Part model, mm, in its own coordinate system. Face numbers are marked on the shaded views. A direction names the side the tool comes from. Give positions to 0.01 mm unless a question says otherwise; leave off trailing zeros. Loops run counter-clockwise (first coordinate to the right, second up) from the corner with the lowest first, then second, coordinate; pieces in that order, holes last. Notation, with made-up numbers: M -35.75,-35 L 8.25,-35 A20 ccw 8.25,-28 Z; hole C 17.25,89 d2. An arc over 180 degrees is marked long. Put each result on its own line as item: value. Start each with the question number.
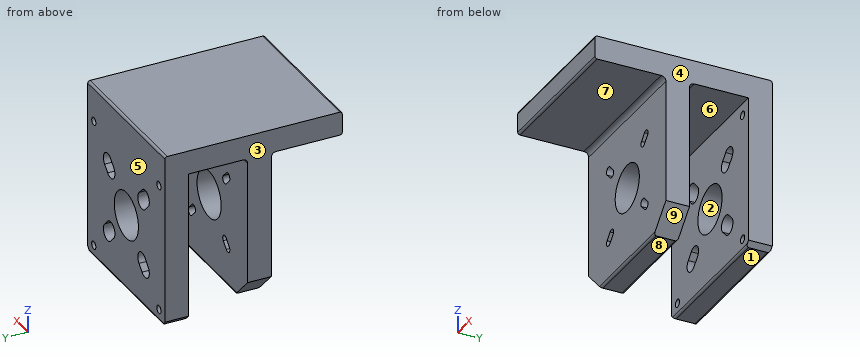
```python
from build123d import *

# Parameters (mm, degrees)
SKETCH_W        = 64
SKETCH_H        = 64
SKETCH_R        = 10
SKETCH_R_2      = 1.7
PAD_DEPTH       = 10
SKETCH001_W     = 64
SKETCH001_H     = 35
PAD001_DEPTH    = 10
SKETCH002_W     = 64
SKETCH002_H     = 74
SKETCH002_R     = 10
PAD002_DEPTH    = 10
SKETCH003_W     = 64
SKETCH003_H     = 10
PAD003_DEPTH    = 30
CHAMFER_SIZE    = 2
CHAMFER001_SIZE = 10
FILLET_R        = 2
FILLET001_R     = 1


with BuildPart() as part:
    # Sketch → Pad (new body)
    with BuildSketch(Plane.XZ):
        Rectangle(SKETCH_W, SKETCH_H)
        Circle(SKETCH_R, mode=Mode.SUBTRACT)
        with Locations((27, 27)):
            Circle(SKETCH_R_2, mode=Mode.SUBTRACT)
        with Locations((-27, -27)):
            Circle(SKETCH_R_2, mode=Mode.SUBTRACT)
        with Locations((-27, 27)):
            Circle(SKETCH_R_2, mode=Mode.SUBTRACT)
        with Locations((27, -27)):
            Circle(SKETCH_R_2, mode=Mode.SUBTRACT)
        with BuildLine():
            ThreePointArc((10.525126, 15.474874), (10.525126, 10.525126), (15.474874, 10.525126))
            Line((17.974874, 13.025126), (15.474874, 10.525126))
            ThreePointArc((17.974874, 13.025126), (17.974874, 17.974874), (13.025126, 17.974874))
            Line((13.025126, 17.974874), (10.525126, 15.474874))
        make_face(mode=Mode.SUBTRACT)
        with BuildLine():
            ThreePointArc((-13.025126, 17.974874), (-17.974874, 17.974874), (-17.974874, 13.025126))
            Line((-15.474874, 10.525126), (-17.974874, 13.025126))
            ThreePointArc((-15.474874, 10.525126), (-10.525126, 10.525126), (-10.525126, 15.474874))
            Line((-10.525126, 15.474874), (-13.025126, 17.974874))
        make_face(mode=Mode.SUBTRACT)
        with BuildLine():
            ThreePointArc((13.025126, -17.974874), (17.974874, -17.974874), (17.974874, -13.025126))
            Line((15.474874, -10.525126), (17.974874, -13.025126))
            ThreePointArc((15.474874, -10.525126), (10.525126, -10.525126), (10.525126, -15.474874))
            Line((10.525126, -15.474874), (13.025126, -17.974874))
        make_face(mode=Mode.SUBTRACT)
        with BuildLine():
            ThreePointArc((-17.974874, -13.025126), (-17.974874, -17.974874), (-13.025126, -17.974874))
            Line((-10.525126, -15.474874), (-13.025126, -17.974874))
            ThreePointArc((-10.525126, -15.474874), (-10.525126, -10.525126), (-15.474874, -10.525126))
            Line((-15.474874, -10.525126), (-17.974874, -13.025126))
        make_face(mode=Mode.SUBTRACT)
    extrude(amount=PAD_DEPTH)

    # Sketch001 (on Face3 of Pad) → Pad001 (join)
    with BuildSketch(Plane(origin=(0, 0, 32), x_dir=(-1, 0, 0), z_dir=(0, 0, 1))):
        with Locations((0, 17.5)):
            Rectangle(SKETCH001_W, SKETCH001_H)
    extrude(amount=PAD001_DEPTH)

    # Sketch002 (on Face31 of Pad001) → Pad002 (join)
    with BuildSketch(Plane.XZ.offset(35)):
        with Locations((0, 5)):
            Rectangle(SKETCH002_W, SKETCH002_H)
        Circle(SKETCH002_R, mode=Mode.SUBTRACT)
        with BuildLine():
            ThreePointArc((11.797918, 14.202082), (11.797918, 11.797918), (14.202082, 11.797918))
            Line((16.702082, 14.297918), (14.202082, 11.797918))
            ThreePointArc((16.702082, 14.297918), (16.702082, 16.702082), (14.297918, 16.702082))
            Line((14.297918, 16.702082), (11.797918, 14.202082))
        make_face(mode=Mode.SUBTRACT)
        with BuildLine():
            ThreePointArc((14.297918, -16.702082), (16.702082, -16.702082), (16.702082, -14.297918))
            Line((14.202082, -11.797918), (16.702082, -14.297918))
            ThreePointArc((14.202082, -11.797918), (11.797918, -11.797918), (11.797918, -14.202082))
            Line((11.797918, -14.202082), (14.297918, -16.702082))
        make_face(mode=Mode.SUBTRACT)
        with BuildLine():
            ThreePointArc((-14.297918, 16.702082), (-16.702082, 16.702082), (-16.702082, 14.297918))
            Line((-14.202082, 11.797918), (-16.702082, 14.297918))
            ThreePointArc((-14.202082, 11.797918), (-11.797918, 11.797918), (-11.797918, 14.202082))
            Line((-11.797918, 14.202082), (-14.297918, 16.702082))
        make_face(mode=Mode.SUBTRACT)
        with BuildLine():
            ThreePointArc((-16.702082, -14.297918), (-16.702082, -16.702082), (-14.297918, -16.702082))
            Line((-11.797918, -14.202082), (-14.297918, -16.702082))
            ThreePointArc((-11.797918, -14.202082), (-11.797918, -11.797918), (-14.202082, -11.797918))
            Line((-14.202082, -11.797918), (-16.702082, -14.297918))
        make_face(mode=Mode.SUBTRACT)
    extrude(amount=PAD002_DEPTH)

    # Sketch003 (on Face37 of Pad002) → Pad003 (join)
    with BuildSketch(Plane.XZ.offset(45)):
        with Locations((0, 37)):
            Rectangle(SKETCH003_W, SKETCH003_H)
    extrude(amount=PAD003_DEPTH)

    # Chamfer
    chamfer_edges = [part.edges().sort_by_distance(p)[0] for p in [
        (32, -5, -32),
        (-32, -5, -32),
    ]]
    chamfer(chamfer_edges, length=CHAMFER_SIZE)

    # Chamfer001
    chamfer001_edges = [part.edges().sort_by_distance(p)[0] for p in [
        (-32, -40, -32),
        (32, -40, -32),
    ]]
    chamfer(chamfer001_edges, length=CHAMFER001_SIZE)

    # Fillet
    fillet_edges = [part.edges().sort_by_distance(p)[0] for p in [
        (0, -35, 32),
        (0, -45, 32),
    ]]
    fillet(fillet_edges, radius=FILLET_R)

    # Fillet001
    fillet001_edges = [part.edges().sort_by_distance(p)[0] for p in [
        (0, -75, 42),
        (0, -75, 32),
        (0, 0, 42),
        (0, -35, -32),
        (0, 0, -32),
        (0, -45, -32),
        (0, -10, -32),
    ]]
    fillet(fillet001_edges, radius=FILLET001_R)


solid = part.part
```
1) Band-saw the part on C-C on z = 31. Give the cut face in (x, y), then the cut area to 3 significant figures.
2) Which spindle directions (+Z, -Z, +X, -X, +Y, -Y) get a long thin tool onto all of the face, cutting with end or side? Do the marked faces 5, 6, 7, 8 and 9. Say none if no direction does.
3) Wall check: L1, parallel to Z at x = -27, y = -4; L2, parallel to Z at x = 0, y = -5.75; L3, parallel to Y at x = -17, z = 22. Give the ranges that are in metal, low to high.
4) Band-saw the part on A-A on z = 0. Give the cut face in (x, y), then the cut area to 3 significant figures.
5) Band-saw the part on B-B on x = 27. Give the cut face in (y, z), then the cut area to 3 significant figures.
6) Mould opens along X. For the marked faces 1, 2, 3 and 4 say: +X half, -X half, draft (parallel to the pull), parting line (faces both ways), or undercut.
7) Band-saw the part on D-D on y = -16. Give the cut face in (x, z).
8) Pin check, flat tips, straight feed: pin 1 Ø23 at (x, z) = (0, 0) entering from -Y; pin 2 Ø2 at (x, z) = (-27, 27) entering from +Y; pin 3 Ø18.5 at (x, y) = (-6.5, -23) entering from -Z. Stop position of each tip, or through.
Evaluation:
1. outline: M -32,-45.27 L 32,-45.27 L 32,-34.73 L -32,-34.73 Z; M -32,-10 L 32,-10 L 32,0 L -32,0 Z
1. area: 1,310 mm2
2. face 5: +Z, -Z, +X, -X, +Y
2. face 6: -Z, +X, -X
2. face 7: -Z, +X, -X, -Y
2. face 8: -Z, +X, -X, +Y, -Y
2. face 9: -Z, +X, -Y
3. L1: -32 to -28.7, -25.3 to 25.3, 28.7 to 42
3. L2: -32 to -10, 10 to 42
3. L3: -45 to -35, -10 to 0
4. outline: M -32,-45 L -10,-45 L -10,-35 L -32,-35 Z; M -32,-10 L -10,-10 L -10,0 L -32,0 Z; M 10,-45 L 32,-45 L 32,-35 L 10,-35 Z; M 10,-10 L 32,-10 L 32,0 L 10,0 Z
4. area: 880 mm2
5. outline: M -75,33 A1 ccw -74,32 L -47,32 A2 cw -45,30 L -45,-27 L -35,-27 L -35,30 A2 cw -33,32 L -10,32 L -10,28.7 L 0,28.7 L 0,41 A1 ccw -1,42 L -74,42 A1 ccw -75,41 Z; M -10,-31 A1 ccw -9,-32 L -1,-32 A1 ccw 0,-31 L 0,-28.7 L -10,-28.7 Z; M -10,-25.3 L 0,-25.3 L 0,25.3 L -10,25.3 Z
5. area: 1,910 mm2
6. face 1: draft
6. face 2: undercut
6. face 3: -X half
6. face 4: +X half
7. outline: M -32,32 L 32,32 L 32,42 L -32,42 Z
8. pin 1: y = -45
8. pin 2: y = -35
8. pin 3: z = 32
